Check sheet for the modelled part. Datum: model origin and axes. Units: mm. Face numbers are marked on the shaded views. A direction names the side the tool comes from. Coordinates: 2 decimals unless noted, no trailing zeros. Loops run counter-clockwise (first coordinate to the right, second up) from the corner with the lowest first, then second, coordinate; pieces in that order, holes last.
```python
from build123d import *

# Parameters (mm, degrees)
SKETCH1_R           = 1.75
BOSS_EXTRUDE1_DEPTH = 6.35
SKETCH5_W           = 20.85
SKETCH5_H           = 14.732
BOSS_EXTRUDE2_DEPTH = 12.7
SKETCH2_R           = 1.125
CUT_EXTRUDE1_DEPTH  = 53.837699391
SKETCH3_R           = 2
CUT_EXTRUDE2_DEPTH  = 11.2
FILLET1_R           = 2.54
FILLET2_R           = 2.54
SKETCH6_R           = 7
CUT_EXTRUDE3_DEPTH  = 53.837699527


with BuildPart() as part:
    # Sketch1 → Boss-Extrude1 (new, symmetric)
    with BuildSketch(Plane(origin=(0, 0, 0), x_dir=(1, 0, 0), z_dir=(0, 1, 0))):
        Polygon((-31.35, -25.859994), (-31.35, 25.859994), (31.35, 25.859994), (31.35, -25.859994), (10.5, -25.859994), (10.5, 18.239994), (-10.5, 18.239994), (-10.5, -25.859994), align=None)
        with Locations(Location((-25, -19.860006, 0), (0, 0, 270))):
            Circle(SKETCH1_R, mode=Mode.SUBTRACT)
        with Locations(Location((25, -19.860006, 0), (0, 0, 270))):
            Circle(SKETCH1_R, mode=Mode.SUBTRACT)
    extrude(amount=BOSS_EXTRUDE1_DEPTH, both=True)

    # Sketch5 → Boss-Extrude2 (add, through all)
    with BuildSketch(Plane.XZ.offset(6.35)):
        with Locations((-20.925, -33.225994)):
            Rectangle(SKETCH5_W, SKETCH5_H)
    extrude(amount=-BOSS_EXTRUDE2_DEPTH)

    # Sketch2 → Cut-Extrude1 (cut, through all)
    with BuildSketch(Plane(origin=(0, 6.35, 0), x_dir=(1, 0, 0), z_dir=(0, 1, 0))):
        with Locations(Location((-28.425, 17.731994, 0), (0, 0, 270))):
            Circle(SKETCH2_R)
        with Locations(Location((-13.425, 17.731994, 0), (0, 0, 270))):
            Circle(SKETCH2_R)
        with Locations(Location((-13.425, 2.731994, 0), (0, 0, 270))):
            Circle(SKETCH2_R)
        with Locations(Location((-28.425, 2.731994, 0), (0, 0, 270))):
            Circle(SKETCH2_R)
        with Locations(Location((-13.425, 37.731994, 0), (0, 0, 270))):
            Circle(SKETCH2_R)
        with Locations(Location((-28.425, 37.731994, 0), (0, 0, 270))):
            Circle(SKETCH2_R)
    extrude(amount=-CUT_EXTRUDE1_DEPTH, mode=Mode.SUBTRACT)

    # Sketch3 → Cut-Extrude2 (cut)
    with BuildSketch(Plane(origin=(0, 6.35, 0), x_dir=(1, 0, 0), z_dir=(0, 1, 0))):
        with Locations(Location((-28.425, 17.731994, 0), (0, 0, 270))):
            Circle(SKETCH3_R)
        with Locations(Location((-13.425, 17.731994, 0), (0, 0, 270))):
            Circle(SKETCH3_R)
        with Locations(Location((-13.425, 2.731994, 0), (0, 0, 270))):
            Circle(SKETCH3_R)
        with Locations(Location((-28.425, 2.731994, 0), (0, 0, 270))):
            Circle(SKETCH3_R)
        with Locations(Location((-28.425, 37.731994, 0), (0, 0, 270))):
            Circle(SKETCH3_R)
        with Locations(Location((-13.425, 37.731994, 0), (0, 0, 270))):
            Circle(SKETCH3_R)
    extrude(amount=-CUT_EXTRUDE2_DEPTH, mode=Mode.SUBTRACT)

    # Fillet1
    # the kernel refuses this fillet: 2.54 mm, written as the material it adds along each edge
    with BuildSketch(Plane(origin=(-10.5, -6.35, -25.859994), x_dir=(0, 0, -1), z_dir=(0, 1, 0))) as fillet1_piece_1:
        with BuildLine():
            CenterArc((FILLET1_R, -FILLET1_R), FILLET1_R, 90, 90)
            Line((0, -FILLET1_R), (0, 0))
            Line((0, 0), (FILLET1_R, 0))
        make_face()
    extrude(amount=12.7)
    # the kernel refuses this fillet: 2.54 mm, written as the material it takes off along each edge
    with BuildSketch(Plane(origin=(-31.35, -12.7, 25.859994), x_dir=(0, 0, -1), z_dir=(0, 1, 0)), Plane(origin=(31.35, 12.7, -25.859994), x_dir=(-1, 0, 0), z_dir=(0, -1, 0)), Plane(origin=(31.35, 12.7, 25.859994), x_dir=(0, 0, -1), z_dir=(0, -1, 0)), Plane(origin=(-10.5, -12.7, 25.859994), x_dir=(-1, 0, 0), z_dir=(0, 1, 0))) as fillet1_2_piece_1:
        with BuildLine():
            CenterArc((FILLET1_R, -FILLET1_R), FILLET1_R, 90, 90)
            Line((0, -FILLET1_R), (0, 0))
            Line((0, 0), (FILLET1_R, 0))
        make_face()
    extrude(amount=25.4, mode=Mode.SUBTRACT)
    with BuildSketch(Plane(origin=(10.5, 12.7, 25.859994), x_dir=(0, 0, -1), z_dir=(0, -1, 0)), Plane(origin=(-31.35, -12.7, -40.591994), x_dir=(0, 0, 1), z_dir=(0, 1, 0)), Plane(origin=(-10.5, -12.7, -40.591994), x_dir=(-1, 0, 0), z_dir=(0, 1, 0))) as fillet1_2_piece_2:
        with BuildLine():
            CenterArc((FILLET1_R, FILLET1_R), FILLET1_R, 180, 90)
            Line((0, FILLET1_R), (0, 0))
            Line((0, 0), (FILLET1_R, 0))
        make_face()
    extrude(amount=25.4, mode=Mode.SUBTRACT)
    with BuildSketch(Plane(origin=(-7.96, 6.35, -25.859994), x_dir=(0, 0, 1), z_dir=(1, 0, 0))) as fillet1_2_piece_3:
        with BuildLine():
            CenterArc((FILLET1_R, FILLET1_R), FILLET1_R, 180, 90)
            Line((0, FILLET1_R), (0, 0))
            Line((0, 0), (FILLET1_R, 0))
        make_face()
    extrude(amount=45.66, mode=Mode.SUBTRACT)
    with BuildSketch(Plane(origin=(-10.5, 6.35, -28.399994), x_dir=(-1, 0, 0), z_dir=(0, 0, -1))) as fillet1_2_piece_4:
        with BuildLine():
            CenterArc((FILLET1_R, -FILLET1_R), FILLET1_R, 90, 90)
            Line((0, -FILLET1_R), (0, 0))
            Line((0, 0), (FILLET1_R, 0))
        make_face()
    extrude(amount=18.542, mode=Mode.SUBTRACT)
    with BuildSketch(Plane(origin=(-7.96, 6.35, -28.399994), x_dir=(-1, 0, 0), z_dir=(0, 0, -1))) as fillet1_2_piece_5:
        with BuildLine():
            CenterArc((2.54 + FILLET1_R, -FILLET1_R), FILLET1_R, 90, 90)
            Line((2.54, -FILLET1_R), (2.54, 0))
            Line((2.54, 0), (2.54 + FILLET1_R, 0))
        make_face()
    revolve(axis=Axis((-7.96, 6.35, -28.399994), (0, 1, 0)), revolution_arc=90, mode=Mode.SUBTRACT)

    # Fillet2
    # the kernel refuses this fillet: 2.54 mm, written as the material it takes off along each edge
    with BuildSketch(Plane(origin=(-6.69, 6.35, -40.591994), x_dir=(0, -1, 0), z_dir=(-1, 0, 0))) as fillet2_piece_1:
        with BuildLine():
            CenterArc((FILLET2_R, FILLET2_R), FILLET2_R, 180, 90)
            Line((0, FILLET2_R), (0, 0))
            Line((0, 0), (FILLET2_R, 0))
        make_face()
    extrude(amount=28.47, mode=Mode.SUBTRACT)

    # Sketch6 → Cut-Extrude3 (cut, through all)
    with BuildSketch(Plane(origin=(0, 6.35, 0), x_dir=(1, 0, 0), z_dir=(0, 1, 0))):
        with Locations(Location((-20.925, 30.231994, 0), (0, 0, 270))):
            Circle(SKETCH6_R)
    extrude(amount=-CUT_EXTRUDE3_DEPTH, mode=Mode.SUBTRACT)


solid = part.part
```
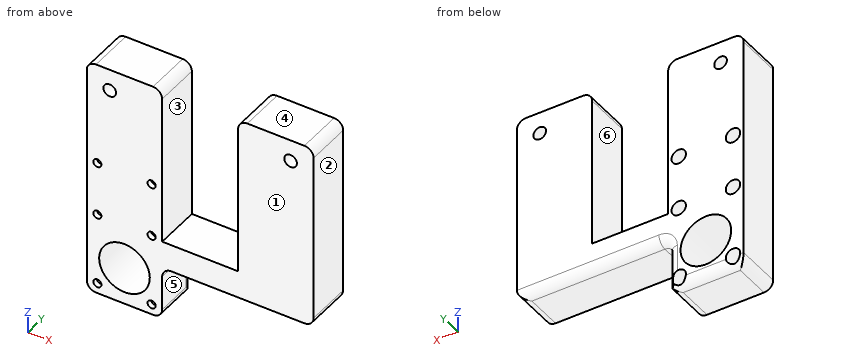
1) Depth check by flat-ended pin: pin 1 (4.5 mm diameter, centred on x = -13, z = -2, fed in from +Y); pin 2 (2 mm diameter, centred on x = -28.5, z = -3, fed in from +Y). Enter the tip coordinate at first touch or a pass-through.
Answer sheet:
pin 1: stops at y = 6.35
pin 2: stops at y = -4.85
2) Scan lines: line 1 (X direction, y = -4.5, z = -13.5); line 2 (Z direction, x = -14.5, y = 0); line 3 (X direction, y = -3.5, z = -38). Record each from-to range of solid material in increasing order.
Answer sheet:
line 1: x = -31.35 to -10.5, 10.5 to 31.35
line 2: z = -40.59 to -39.42, -36.05 to -33.01, -27.45 to -19.42, -16.05 to -4.42, -1.05 to 25.86
line 3: x = -31.35 to -30.41, -26.44 to -15.41, -11.44 to -10.5
3) Set-up check for the marked faces 4, 5 and 6: record each of +Z, -Z, +X, -X, +Y, -Y from which the full face is reachable in a straight line by a thin tool's end or side.
Answer sheet:
face 4: +Z, +X, -X, +Y, -Y
face 5: -Z, +X, +Y, -Y
face 6: +Z, +Y, -Y
4) Section check A-A on x = 25. Enter the section's corners in (y, z), plus the area to 3 significant figures.
Answer sheet:
outline: (-6.35, -25.86) - (3.81, -25.86) arc R2.54 ccw to (6.35, -23.32) - (6.35, 18.11) - (-6.35, 18.11) - close; (-6.35, 21.61) - (6.35, 21.61) - (6.35, 25.86) - (-6.35, 25.86) - close
area: 611 mm2
5) Section check C-C on x = -24. Enter the section's corners in (y, z).
Answer sheet:
outline: (-6.35, -40.59) - (3.81, -40.59) arc R2.54 ccw to (6.35, -38.05) - (6.35, -36.52) - (-6.35, -36.52) - close; (-6.35, -23.94) - (6.35, -23.94) - (6.35, 18.42) - (-6.35, 18.42) - close; (-6.35, 21.3) - (6.35, 21.3) - (6.35, 25.86) - (-6.35, 25.86) - close
6) Mould release check, pull along X, two halves, no side actions. Record for the marked faces 1, 2 and 3: +X half, -X half, draft (parallel to the pull), parting line (faces both ways), or undercut.
Answer sheet:
face 1: draft
face 2: +X half
face 3: undercut
7) Section check B-B on z = 1.5. Enter the section's corners in (x, y).
Answer sheet:
outline: (-31.35, -6.35) - (-10.5, -6.35) - (-10.5, 6.35) - (-31.35, 6.35) - close; (10.5, -6.35) - (31.35, -6.35) - (31.35, 6.35) - (10.5, 6.35) - close
8) Section check D-D on y = -3.25. Give the number of separate pieces and of enclosed holes in the cut face, plus the area to 3 significant figures.
Answer sheet:
separate pieces: 1
enclosed holes: 9
area: 2,370 mm2
